Can you work these out from the drawing? Everything is in mm from the part's minimum corner. Coordinates: 2 decimals unless noted, no trailing zeros. Loops run counter-clockwise (first coordinate to the right, second up) from the corner with the lowest first, then second, coordinate; pieces in that order, holes last.
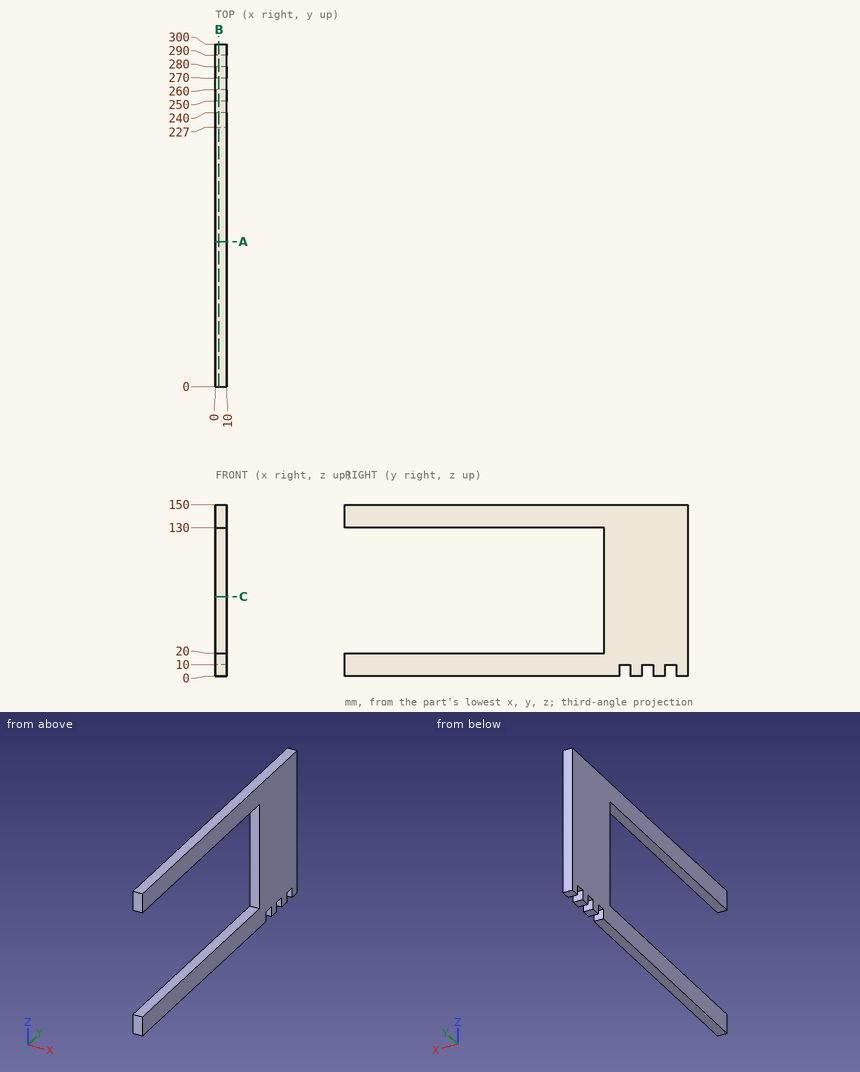
Item 1: I need wall thicknesses on line 1 along Z through (x, y) = (8.25, 127); line 2 along Y through (x, z) = (3.25, 7); line 3 along Y through (x, z) = (3.5, 31). Which ranges of each line are inside material? Lowest first, please.
Results are:
line 1: z = 0 to 20, 130 to 150
line 2: y = 0 to 240, 250 to 260, 270 to 280, 290 to 300
line 3: y = 227 to 300
Item 2: Suppose I cut it at C-C, the plane z = 69.5. Please give me the cut outline in (x, y).
Results are:
outline: (0, 227) - (10, 227) - (10, 300) - (0, 300) - close
Item 3: Suppose I cut it at A-A, the plane y = 127. Please give me the cut outline in (x, z), plus the area to 3 significant figures.
Results are:
outline: (0, 0) - (10, 0) - (10, 20) - (0, 20) - close; (0, 130) - (10, 130) - (10, 150) - (0, 150) - close
area: 400 mm2
Item 4: I'm going to push flat-ended pins straight in: P1, Ø3, axis at x = 6, y = 267, coming from the -Z side; P2, Ø1, axis at x = 5.5, z = 124, coming from the -Y side. Where does each tip first touch, or does it pass through?
Results are:
P1: stops at z = 10
P2: stops at y = 227
Item 5: Suppose I cut it at B-B, the plane x = 3. Please give me the cut outline in (y, z).
Results are:
outline: (0, 0) - (240, 0) - (240, 10) - (250, 10) - (250, 0) - (260, 0) - (260, 10) - (270, 10) - (270, 0) - (280, 0) - (280, 10) - (290, 10) - (290, 0) - (300, 0) - (300, 150) - (0, 150) - (0, 130) - (227, 130) - (227, 20) - (0, 20) - close
